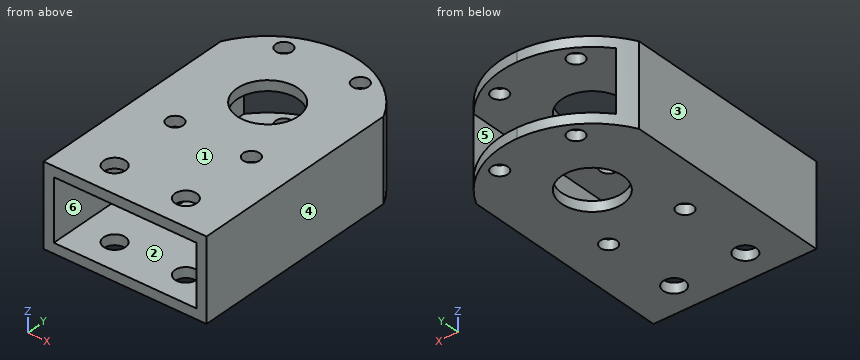
from build123d import *

# Parameters (mm, degrees)
SKETCH1_W               = 50.8
SKETCH1_H               = 25.4
SKETCH1_W_2             = 44.45
SKETCH1_H_2             = 19.05
EXTRUDE_THIN1_DEPTH     = 82.55
F_10_CLEARANCE_HOLE1_D  = 5.1054
SKETCH7_R               = 9.525
CUT_EXTRUDE2_DEPTH      = 1
CUT_EXTRUDE2_DEPTH_BACK = 26.4
F_1_4_CLEARANCE_HOLE2_D = 6.7564
CUT_EXTRUDE3_DEPTH      = 26.4


with BuildPart() as part:
    # Sketch1 → Extrude-Thin1 (new body)
    with BuildSketch(Plane(origin=(0, 0, 0), x_dir=(1, 0, 0), z_dir=(0, 1, 0))):
        Rectangle(SKETCH1_W, SKETCH1_H)
        Rectangle(SKETCH1_W_2, SKETCH1_H_2, mode=Mode.SUBTRACT)
    extrude(amount=EXTRUDE_THIN1_DEPTH)

    # #10 Clearance Hole1 (through all)
    with Locations(Plane(origin=(0, 0, -12.7), x_dir=(-1, 0, 0), z_dir=(0, 0, -1))):
        with Locations((-11.90625, 33.352770072), (-11.90625, 74.597229928), (11.90625, 74.597229928), (11.90625, 33.352770072)):
            Hole(F_10_CLEARANCE_HOLE1_D / 2)

    # Sketch7 → Cut-Extrude2 (cut, two sides)
    with BuildSketch(Plane(origin=(0, 0, -12.7), x_dir=(-1, 0, 0), z_dir=(0, 0, -1))) as cut_extrude2_sk:
        with Locations((0, 53.975)):
            Circle(SKETCH7_R)
    extrude(amount=CUT_EXTRUDE2_DEPTH, mode=Mode.SUBTRACT)
    extrude(cut_extrude2_sk.sketch, amount=-CUT_EXTRUDE2_DEPTH_BACK, mode=Mode.SUBTRACT)

    # 1/4 Clearance Hole2 (through all)
    with Locations(Plane.XY.offset(12.7)):
        with Locations((-11.1125, 9.525), (11.1125, 9.525), (-109.171479686, 68.785430569)):
            Hole(F_1_4_CLEARANCE_HOLE2_D / 2)

    # Sketch10 → Cut-Extrude3 (cut, through all)
    with BuildSketch(Plane(origin=(0, 0, -12.7), x_dir=(-1, 0, 0), z_dir=(0, 0, -1))):
        with BuildLine():
            Line((-25.4, 82.55), (-25.4, 67.065860361))
            ThreePointArc((-25.4, 67.065860361), (-14.873790542, 78.373790542), (0, 82.55))
            Line((0, 82.55), (-25.4, 82.55))
        make_face()
        with BuildLine():
            Line((25.4, 82.55), (0, 82.55))
            ThreePointArc((0, 82.55), (14.873790542, 78.373790542), (25.4, 67.065860361))
            Line((25.4, 67.065860361), (25.4, 82.55))
        make_face()
    extrude(amount=-CUT_EXTRUDE3_DEPTH, mode=Mode.SUBTRACT)


solid = part.part
Geometry: final body of the model. Coordinates: model frame, mm. Face numbers are marked on the shaded views. A direction names the side the tool comes from. Coordinates: 2 decimals unless noted, no trailing zeros. Loops run counter-clockwise (first coordinate to the right, second up) from the corner with the lowest first, then second, coordinate; pieces in that order, holes last. Notation, with made-up numbers: (17, -0.5) - (47, -0.5) arc R28 cw to (47, 29.5) - close; hole circle Ø8 at (-27, 69). An arc over 180 degrees is marked (long way). Put each result on its own line as item: value. Start each with the question number.
Q1. Set-up query: the marked faces 1 and 2. Return all of +Z, -Z, +X, -X, +Y, -Y with unobstructed straight access to the full face (end or side cutting, diameter ignored); none if empty.
Q2. Pin query (flat end, axial travel): pin 1 Ø4.5 at (x, y) = (-11.91, 74.6) entering from +Z. Return the tip coordinate at first contact, or that it passes through.
Q3. Line query: line 1 (Z direction, x = 10.5, y = 5) (3 decimals); line 2 (X direction, y = 20, z = 1) (3 decimals); line 3 (Y direction, x = 4.5, z = 11). Output: solid intervals per line, ascending.
Q4. Cut plane B-B, the plane x = -12. Give the number of separate pieces and of enclosed holes in the cut face, and give its area (3 significant figures).
Q5. Cut plane D-D, the plane y = 7.5. Return loops of the section in (x, z) (1 decimal), and give its area (3 significant figures).
Q6. Cut plane C-C, the plane x = 5.5. Return loops of the section in (y, z) (3 decimals), and give its area (3 significant figures).
Q7. Cut plane A-A, the plane z = 5.25. Return loops of the section in (x, y) (3 decimals).
Q8. Pull-direction query (X, two-part tool) for the marked faces 3, 4, 5 and 6; classes: released by +X, released by -X, zero draft, split by the parting line, or undercut.
Filled sheet:
1. face 1: +Z, +X, -X, +Y, -Y
1. face 2: +Y, -Y
2. pin 1: through
3. line 1: -12.7 to -9.525, 9.525 to 12.7
3. line 2: -25.4 to -22.225, 22.225 to 25.4
3. line 3: 0 to 45.58, 62.37 to 82.19
4. separate pieces: 8
4. enclosed holes: 0
4. area: 401 mm²
5. outline: (-25.4, -12.7) - (-13.8, -12.7) - (-13.8, -9.5) - (-22.2, -9.5) - (-22.2, 9.5) - (-13.8, 9.5) - (-13.8, 12.7) - (-25.4, 12.7) - close; (-8.4, -12.7) - (8.4, -12.7) - (8.4, -9.5) - (-8.4, -9.5) - close; (-8.4, 9.5) - (8.4, 9.5) - (8.4, 12.7) - (-8.4, 12.7) - close; (13.8, -12.7) - (25.4, -12.7) - (25.4, 12.7) - (13.8, 12.7) - (13.8, 9.5) - (22.2, 9.5) - (22.2, -9.5) - (13.8, -9.5) - close
5. area: 375 mm²
6. outline: (0, -12.7) - (46.198, -12.7) - (46.198, -9.525) - (0, -9.525) - close; (0, 9.525) - (46.198, 9.525) - (46.198, 12.7) - (0, 12.7) - close; (61.752, -12.7) - (82.016, -12.7) - (82.016, -9.525) - (61.752, -9.525) - close; (61.752, 9.525) - (82.016, 9.525) - (82.016, 12.7) - (61.752, 12.7) - close
6. area: 422 mm²
7. outline: (-25.4, 0) - (-22.225, 0) - (-22.225, 71.936) arc R28.575 ccw to (-25.4, 67.066) - close; (22.225, 0) - (25.4, 0) - (25.4, 67.066) arc R28.575 ccw to (22.225, 71.936) - close
8. face 3: released by -X
8. face 4: released by +X
8. face 5: undercut
8. face 6: undercut
